Part model, mm, in its own coordinate system. Face numbers are marked on the shaded views. A direction names the side the tool comes from. Round coordinates to 2 decimals unless told otherwise and drop trailing zeros. Loops run counter-clockwise (first coordinate to the right, second up) from the corner with the lowest first, then second, coordinate; pieces in that order, holes last. Notation, with made-up numbers: (10, 37) - (34, 37) arc R29 cw to (34, 70) - close; hole circle Ø8 at (-8, -1). An arc over 180 degrees is marked (long way). Write each question's results on one line, items separated by ' | '. Start each with the question number.
(1) Tool access for the marked faces 5, 6, 7, 8 and 9: list every direction of +Z, -Z, +X, -X, +Y, -Y with a clear straight run to the whole face (end or side of a thin tool).
(2) Flat gauge pins, fed straight in: P1, Ø18, axis at x = -14, y = 10, coming from the -Z side; P2, Ø18, axis at y = 9, z = -16, coming from the -X side; P3, Ø1.3, axis at y = 25, z = -11.5, coming from the -X side; P4, Ø6, axis at y = 28, z = 8.5, coming from the +X side. Where does each tip first touch, or does it go through?
(3) Cut at A-A, the plane x = -18.5. List the corners of the cut face in (y, z), then the cut area to 3 significant figures.
(4) Mould opens along Y. For the marked faces 1, 2, 3 and 4 say: released by +Y, released by -Y, zero draft, split by the parting line, or undercut.
(5) Cut at D-D, the plane z = -14. List the corners of the cut face in (x, y), then the cut area to 3 significant figures.
(6) Cut at C-C, the plane x = -24.13. List the corners of the cut face in (y, z), then the cut area to 3 significant figures.
(7) Drill centre lines: L1, parallel to Z at x = -17.5, y = 11.5; L2, parallel to Y at x = -13, z = -7.5; L3, parallel to X at y = 11.5, z = -20.5. Where is each one in solid material? Low to high.
(8) Cut at B-B, the plane z = -1.5. List the corners of the cut face in (x, y).
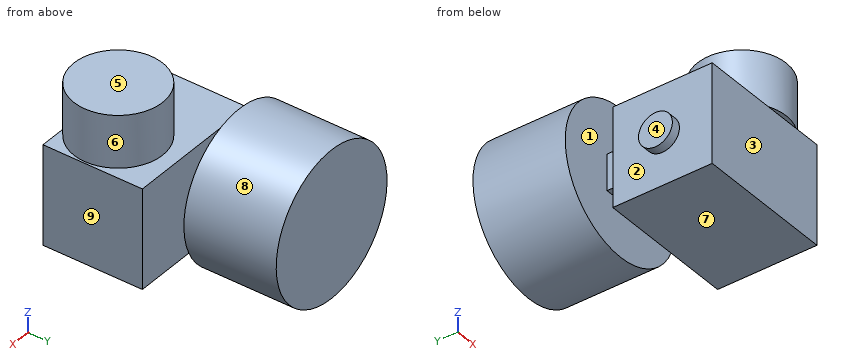
from build123d import *

# Parameters (mm, degrees)
SKETCH1_W           = 22.352
SKETCH1_H           = 22.352
BOSS_EXTRUDE1_DEPTH = 31.242
SKETCH2_R           = 3.81
BOSS_EXTRUDE2_DEPTH = 1.0541
SKETCH3_W           = 8.128
SKETCH3_H           = 8.128
BOSS_EXTRUDE3_DEPTH = 2.54
SKETCH4_R           = 16.5227
BOSS_EXTRUDE4_DEPTH = 20.7518
SKETCH5_R           = 3.81
BOSS_EXTRUDE5_DEPTH = 2.1082
SKETCH6_R           = 6.35
BOSS_EXTRUDE7_DEPTH = 2.54
SKETCH7_R           = 9.9822
BOSS_EXTRUDE8_DEPTH = 11.7348


with BuildPart() as part:
    # Sketch1 → Boss-Extrude1 (new body)
    with BuildSketch(Plane(origin=(0, 0, 0), x_dir=(0, 0, -1), z_dir=(1, 0, 0))):
        with Locations((11.176, 11.176)):
            Rectangle(SKETCH1_W, SKETCH1_H)
    extrude(amount=-BOSS_EXTRUDE1_DEPTH)

    # Sketch2 → Boss-Extrude2 (add)
    with BuildSketch(Plane(origin=(0, 22.352, 0), x_dir=(1, 0, 0), z_dir=(0, 1, 0))):
        with Locations(Location((-24.13, 11.176, 0), (0, 0, 270))):
            Circle(SKETCH2_R)
    extrude(amount=BOSS_EXTRUDE2_DEPTH)

    # Sketch3 → Boss-Extrude3 (add)
    with BuildSketch(Plane(origin=(0, 23.4061, 0), x_dir=(1, 0, 0), z_dir=(0, 1, 0))):
        with Locations((-24.13, 11.176)):
            Rectangle(SKETCH3_W, SKETCH3_H)
    extrude(amount=BOSS_EXTRUDE3_DEPTH)

    # Sketch4 → Boss-Extrude4 (add)
    with BuildSketch(Plane(origin=(0, 25.9461, 0), x_dir=(1, 0, 0), z_dir=(0, 1, 0))):
        with Locations(Location((-24.13, 11.176, 0), (0, 0, 90))):
            Circle(SKETCH4_R)
    extrude(amount=BOSS_EXTRUDE4_DEPTH)

    # Sketch5 → Boss-Extrude5 (add)
    with BuildSketch(Plane.ZY.offset(31.242)):
        with Locations((-11.176, 11.176)):
            Circle(SKETCH5_R)
    extrude(amount=BOSS_EXTRUDE5_DEPTH)

    # Sketch6 → Boss-Extrude7 (add)
    with BuildSketch(Plane.XY):
        with Locations((-7.62, 11.176)):
            Circle(SKETCH6_R)
    extrude(amount=BOSS_EXTRUDE7_DEPTH)

    # Sketch7 → Boss-Extrude8 (add)
    with BuildSketch(Plane.XY.offset(2.54)):
        with Locations((-7.62, 11.176)):
            Circle(SKETCH7_R)
    extrude(amount=BOSS_EXTRUDE8_DEPTH)


solid = part.part
A:
1) face 5: +Z, +X, -X, +Y, -Y | face 6: +Z | face 7: -Z, +X, -X, -Y | face 8: +Y | face 9: -Z, +X, +Y, -Y
2) P1: z = -22.35 | P2: x = -33.35 | P3: x = -28.19 | P4: through
3) outline: (0, -22.35) - (22.35, -22.35) - (22.35, 0) - (0, 0) - close; (25.95, -26.71) - (46.7, -26.71) - (46.7, 4.36) - (25.95, 4.36) - close | area: 1,140 mm2
4) face 1: undercut | face 2: undercut | face 3: released by -Y | face 4: zero draft
5) outline: (-40.41, 25.95) - (-28.19, 25.95) - (-28.19, 23.41) - (-26.69, 23.41) - (-26.69, 22.35) - (-31.24, 22.35) - (-31.24, 13.73) - (-33.35, 13.73) - (-33.35, 8.62) - (-31.24, 8.62) - (-31.24, 0) - (0, 0) - (0, 22.35) - (-21.57, 22.35) - (-21.57, 23.41) - (-20.07, 23.41) - (-20.07, 25.95) - (-7.85, 25.95) - (-7.85, 46.7) - (-40.41, 46.7) - close | area: 1,410 mm2
6) outline: (0, -22.35) - (22.35, -22.35) - (22.35, -14.99) - (23.41, -14.99) - (23.41, -15.24) - (25.95, -15.24) - (25.95, -27.7) - (46.7, -27.7) - (46.7, 5.35) - (25.95, 5.35) - (25.95, -7.11) - (23.41, -7.11) - (23.41, -7.37) - (22.35, -7.37) - (22.35, 0) - (0, 0) - close | area: 1,210 mm2
7) L1: -22.35 to 0, 2.54 to 14.27 | L2: 0 to 22.35, 25.95 to 46.7 | L3: -31.24 to 0
8) outline: (-37.52, 25.95) - (-10.74, 25.95) - (-10.74, 46.7) - (-37.52, 46.7) - close; (-31.24, 0) - (0, 0) - (0, 22.35) - (-31.24, 22.35) - close
